Build history of the part. All positions in model axes, mm. Face numbers are marked on the shaded views. A direction names the side the tool comes from. Coordinates: 2 decimals unless noted, no trailing zeros. Order: outer loops, then holes, each group sorted by start corner. A loop starts at its lowest first (then second) coordinate and runs counter-clockwise, first axis right, second up. Notation, with made-up numbers: (-39, 33) - (-21, 33) arc R22 cw to (-21, 48) - close; hole circle Ø3 at (61, -6.5). An arc over 180 degrees is marked (long way). Return JSON: item names as keys, results as strings.
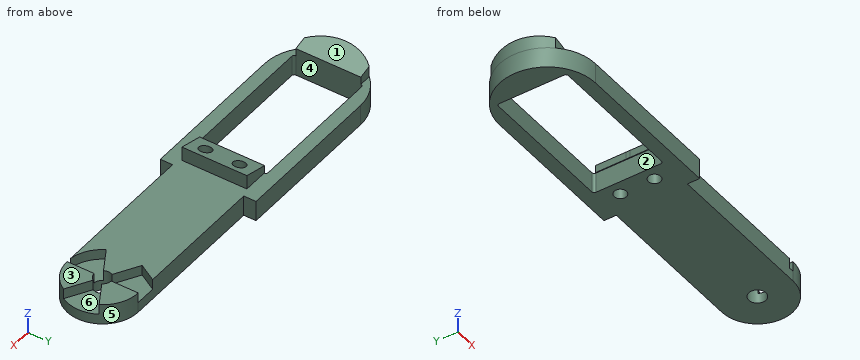
from build123d import *

# Parameters (mm, degrees)
SKETCH1_R            = 2.5
BOSS_EXTRUDE1_DEPTH  = 6
CUT_EXTRUDE4_START   = -3
CUT_EXTRUDE4_DEPTH   = 3
BOSS_EXTRUDE3_START  = -6
BOSS_EXTRUDE3_DEPTH  = 6
BOSS_EXTRUDE4_DEPTH  = 6
CUT_EXTRUDE8_DEPTH   = 216.487496567
BOSS_EXTRUDE5_REACH  = 217.487
M3_CLEARANCE_HOLE2_D = 3.6
BOSS_EXTRUDE6_REACH  = 217.487


with BuildPart() as part:
    # Sketch1 → Boss-Extrude1 (new body)
    with BuildSketch(Plane.XY):
        with BuildLine():
            Line((173.900000276, 87.099556458), (88.800000276, 87.099467009))
            ThreePointArc((88.800000276, 87.099467009), (78.399532162, 97.499935123), (88.800000276, 107.900403236))
            Line((88.800000276, 107.900403236), (173.900000276, 107.900313787))
            ThreePointArc((173.900000276, 107.900313787), (184.30037894, 97.499940589), (173.900000276, 87.099556458))
        make_face()
        with Locations((88.800000276, 97.499935123)):
            Circle(SKETCH1_R, mode=Mode.SUBTRACT)
        with Locations((173.900000276, 97.499935123)):
            Circle(SKETCH1_R, mode=Mode.SUBTRACT)
    extrude(amount=BOSS_EXTRUDE1_DEPTH)

    # Sketch2 → Cut-Extrude4 (cut)
    with BuildSketch(Plane.XY.offset(6).offset(CUT_EXTRUDE4_START)):
        with BuildLine():
            ThreePointArc((176.065063128, 98.749936261), (176.400000276, 97.499936437), (176.065064442, 96.249936261))
            Line((176.065064442, 96.249936261), (182.993597708, 92.24975057))
            ThreePointArc((182.993597708, 92.24975057), (184.40037894, 97.499940641), (182.993592189, 102.750129234))
            Line((182.993592189, 102.750129234), (176.065063128, 98.749936261))
        make_face()
        with BuildLine():
            ThreePointArc((164.806408362, 92.249741011), (168.649815723, 88.406337691), (173.900005794, 86.999556458))
            Line((173.900005794, 86.999556458), (173.90000159, 94.999935123))
            ThreePointArc((173.90000159, 94.999935123), (172.650001414, 95.334870956), (171.734937423, 96.249933985))
            Line((171.734937423, 96.249933985), (164.806408362, 92.249741011))
        make_face()
        with BuildLine():
            Line((173.899998962, 99.999935123), (173.899994757, 108.000313787))
            Line((173.899994757, 108.000313787), (167.779868906, 107.90032022))
            Line((167.779868906, 107.90032022), (164.806402844, 102.750119676))
            Line((164.806402844, 102.750119676), (171.73493611, 98.749933985))
            ThreePointArc((171.73493611, 98.749933985), (172.649999138, 99.664997975), (173.899998962, 99.999935123))
        make_face()
    extrude(amount=CUT_EXTRUDE4_DEPTH, mode=Mode.SUBTRACT)

    # Sketch4 → Boss-Extrude3 (add)
    with BuildSketch(Plane.XY.offset(6).offset(BOSS_EXTRUDE3_START)):
        with BuildLine():
            Line((85.800000276, 107.900403236), (88.800000276, 107.900403236))
            ThreePointArc((88.800000276, 107.900403236), (78.399532162, 97.499935123), (88.800000276, 87.099467009))
            Line((88.800000276, 87.099467009), (85.800000276, 87.099467009))
            ThreePointArc((85.800000276, 87.099467009), (75.399532162, 97.499935123), (85.800000276, 107.900403236))
        make_face()
    extrude(amount=BOSS_EXTRUDE3_DEPTH)

    # Sketch9 → Boss-Extrude4 (add)
    with BuildSketch(Plane.XY.offset(6)):
        with BuildLine():
            Line((85.2774961, 111.499917036), (129.322504452, 111.499917036))
            Line((129.322504452, 111.499917036), (129.322504452, 83.49995321))
            Line((129.322504452, 83.49995321), (85.322504452, 83.49995321))
            ThreePointArc((85.322504452, 83.49995321), (71.300018363, 97.477430947), (85.2774961, 111.499917036))
        make_face()
    extrude(amount=-BOSS_EXTRUDE4_DEPTH)

    # Sketch8 → Cut-Extrude8 (cut, through all)
    with BuildSketch(Plane.XY.offset(6)):
        with BuildLine():
            Line((78.600000246, 87.999935155), (78.600000306, 106.999935155))
            ThreePointArc((78.600000306, 106.999935155), (78.805025561, 107.494909902), (79.300000309, 107.699935153))
            Line((79.300000309, 107.699935153), (118.700000309, 107.699935027))
            ThreePointArc((118.700000309, 107.699935027), (119.194975055, 107.494909772), (119.400000306, 106.999935025))
            Line((119.400000306, 106.999935025), (119.400000246, 87.999935025))
            ThreePointArc((119.400000246, 87.999935025), (119.194974991, 87.504960279), (118.700000243, 87.299935027))
            Line((118.700000243, 87.299935027), (79.300000243, 87.299935153))
            ThreePointArc((79.300000243, 87.299935153), (78.805025497, 87.504960408), (78.600000246, 87.999935155))
        make_face()
    extrude(amount=-CUT_EXTRUDE8_DEPTH, mode=Mode.SUBTRACT)

    # Boss-Extrude5: up to this plane
    boss_extrude5_end = Plane(origin=(125.750000277, 97.974935005, 9.9), z_dir=(-0.2512185729888078, 8.03898804267201e-10, 0.9679303841627594))
    # Sketch13 → Boss-Extrude5 (add, up to the surface)
    with BuildSketch(Plane.XY.offset(6), mode=Mode.PRIVATE) as boss_extrude5_sk1:
        Polygon((119.200000274, 96.924935025), (119.200000246, 87.999935025), (126.700000306, 87.999935025), (126.700000306, 106.999935025), (119.200000306, 106.999935025), (119.200000278, 98.074935025), align=None)
    boss_extrude5_tool1 = split(extrude(boss_extrude5_sk1.sketch, amount=BOSS_EXTRUDE5_REACH, mode=Mode.PRIVATE), bisect_by=boss_extrude5_end, keep=Keep.BOTH, mode=Mode.PRIVATE)
    add(boss_extrude5_tool1.solids().sort_by_distance((122.95, 97.499935, 6))[0])

    # M3 Clearance Hole2 (through all)
    with Locations(Plane(origin=(0, 0, 0), x_dir=(-1, 0, 0), z_dir=(0, 0, -1))):
        with Locations((-123.250000292, 102.499935013), (-123.25000026, 92.499935013)):
            Hole(M3_CLEARANCE_HOLE2_D / 2)

    # Boss-Extrude6: up to this plane
    boss_extrude6_end = Plane(origin=(72.250000277, 97.974935176, 9.9), z_dir=(0.2512185729888078, -8.038995017974768e-10, 0.9679303841627596))
    # Sketch17 → Boss-Extrude6 (add, up to the surface)
    with BuildSketch(Plane.XY.offset(6), mode=Mode.PRIVATE) as boss_extrude6_sk1:
        with BuildLine():
            Line((75.016518346, 87.999935155), (78.600000246, 87.999935155))
            Line((78.600000246, 87.999935155), (78.600000306, 106.999935155))
            Line((78.600000306, 106.999935155), (75.016518405, 106.999935155))
            ThreePointArc((75.016518405, 106.999935155), (71.300000276, 97.499935166), (75.016518346, 87.999935155))
        make_face()
    boss_extrude6_tool1 = split(extrude(boss_extrude6_sk1.sketch, amount=BOSS_EXTRUDE6_REACH, mode=Mode.PRIVATE), bisect_by=boss_extrude6_end, keep=Keep.BOTH, mode=Mode.PRIVATE)
    add(boss_extrude6_tool1.solids().sort_by_distance((75.437055, 97.499935, 6))[0])


solid = part.part
1. Cut at C-C on x = 153. Give the cut face in (y, z), plus the area to 3 significant figures.
Check values:
{"outline": "(87.1, 0) - (107.9, 0) - (107.9, 6) - (87.1, 6) - close", "area": "125 mm²"}
2. Drop flat-ended pins along their axis: pin 1 (6 mm diameter, centred on y = 93.5, z = 5.5, fed in from -X); pin 2 (5 mm diameter, centred on x = 161.5, z = 4, fed in from -Y); pin 3 (1 mm diameter, centred on y = 108, z = 1.5, fed in from -X); pin 4 (3 mm diameter, centred on x = 123.25, y = 92.5, fed in from -Z). Give the stop position or say it passes through.
Check values:
{"pin 1": "x = 71.34", "pin 2": "y = 87.1", "pin 3": "x = 75.5", "pin 4": "through"}
3. Mould opens along X. For the marked faces 4, 5 and 6 say: pulls with the +X half, pulls with the -X half, needs draft (parallel to the pull), parting line crosses it, or undercut.
Check values:
{"face 4": "undercut", "face 5": "pulls with the +X half", "face 6": "needs draft"}
4. Cut at B-B on x = 97. Give the cut face in (y, z).
Check values:
{"outline": "(83.5, 0) - (87.3, 0) - (87.3, 6) - (83.5, 6) - close; (107.7, 0) - (111.5, 0) - (111.5, 6) - (107.7, 6) - close"}
5. Cut at A-A on z = 4.75. State how many separate pieces and enclosed holes the cut face has, plus the area to 3 significant figures.
Check values:
{"separate pieces": "3", "enclosed holes": "3", "area": "1,600 mm²"}
6. Probe L1, parallel to Y at x = 123.25, z = 6.5; L2, parallel to X at y = 88.25, z = 4.5; L3, parallel to Y at x = 123.25, z = 4. List the from-to ranges inside material, lowest first.
Check values:
{"L1": "88 to 90.7, 94.3 to 100.7, 104.3 to 107", "L2": "74.79 to 78.6, 119.4 to 168.93, 173.9 to 178.65", "L3": "83.5 to 90.7, 94.3 to 100.7, 104.3 to 111.5"}
7. Tool access for the marked faces 1, 2 and 3: list every direction of +Z, -Z, +X, -X, +Y, -Y with a clear straight run to the whole face (end or side of a thin tool).
Check values:
{"face 1": "+Z, +Y, -Y", "face 2": "-Z", "face 3": "+Z, +X, +Y, -Y"}
